```python
from build123d import *

# Parameters (mm, degrees)
SKETCH1_W                = 43
SKETCH1_H                = 40
BOSS_EXTRUDE1_DEPTH      = 5.5
FILLET1_R                = 1
SKETCH2_W                = 3
SKETCH2_H                = 5.5
BOSS_EXTRUDE2_DEPTH      = 3
BOSS_EXTRUDE2_DEPTH_BACK = 3


with BuildPart() as part:
    # Sketch1 → Boss-Extrude1 (new body)
    with BuildSketch(Plane(origin=(0, 0, 0), x_dir=(1, 0, 0), z_dir=(0, 1, 0))):
        Rectangle(SKETCH1_W, SKETCH1_H)
    extrude(amount=BOSS_EXTRUDE1_DEPTH)

    # Fillet1
    fillet1_edges = [part.edges().sort_by_distance(p)[0] for p in [
        (0, 5.5, -20),
        (0, 0, -20),
        (0, 0, 20),
        (0, 5.5, 20),
    ]]
    fillet(fillet1_edges, radius=FILLET1_R)

    # Sketch2 → Boss-Extrude2 (add, two sides)
    with BuildSketch(Plane.XY.offset(20)) as boss_extrude2_sk:
        with Locations((-20, 2.75)):
            Rectangle(SKETCH2_W, SKETCH2_H)
    extrude(amount=BOSS_EXTRUDE2_DEPTH)
    extrude(boss_extrude2_sk.sketch, amount=-BOSS_EXTRUDE2_DEPTH_BACK)


solid = part.part
```
Design review of the part built by this model. Coordinates are the model's own, in mm. A direction names the side the tool comes from. Round coordinates to 2 decimals unless told otherwise and drop trailing zeros. Write each loop counter-clockwise with the first axis right and the second up, starting at its lowest first coordinate (ties: lowest second). Pieces come first, ordered by that corner, then holes. Notation, with made-up numbers: (-38, -30) -> (-20, -30) arc R21 ccw to (-20, -2) -> close; hole circle Ø3 at (10, 6.5). An arc over 180 degrees is marked (long way). Answer in a Markdown table with one row per item.
Q1. For faces 1 (the face through (0, 3, -20)), 2 (the face through (0, 5.5, 2)), 3 (the face through (1, 3, 20)), 4 (the face through (1.78, 5.199, 19.715)), 5 (the face through (1.78, 0.301, 19.715)), list the 3-axis set-ups (+Z, -Z, +X, -X, +Y, -Y) from which the entire face can be reached by the end or side of a thin tool; tool diameter is ignored.
The answers:
| item | result |
|---|---|
| face 1 | -Z, +X, -X, +Y, -Y |
| face 2 | +Z, -Z, +X, -X, +Y |
| face 3 | +Z, +X, +Y, -Y |
| face 4 | +Z, +X, +Y |
| face 5 | +Z, +X, -Y |
Q2. Take a section at B-B, the plane y = 2.25. State the section outline as (x, z) points.
The answers:
| item | result |
|---|---|
| outline | (-21.5, -20) -> (21.5, -20) -> (21.5, 20) -> (-18.5, 20) -> (-18.5, 23) -> (-21.5, 23) -> close |
Q3. Take a section at A-A, the plane x = -8. State the section outline as (y, z) points, then the cut area to 3 significant figures.
The answers:
| item | result |
|---|---|
| outline | (0, -19) arc R1 ccw to (1, -20) -> (4.5, -20) arc R1 ccw to (5.5, -19) -> (5.5, 19) arc R1 ccw to (4.5, 20) -> (1, 20) arc R1 ccw to (0, 19) -> close |
| area | 219 mm² |
Q4. To check wall thickness, follow L1, parallel to Z at x = 16.5, y = 3.55; L2, parallel to Z at x = -16, y = 0.6. State the ranges of each line that lie inside material, in increasing order. Write a range as [from, to].
The answers:
| item | result |
|---|---|
| L1 | [-20, 20] |
| L2 | [-19.92, 19.92] |
Q5. Clearance check with a flat-ended pin moving along its axis: pin 1 Ø1.5 at (x, y) = (9, 0.5) entering from +Z. State where the tip first meets the part, or that it passes through.
The answers:
| item | result |
|---|---|
| pin 1 | z = 20 |
